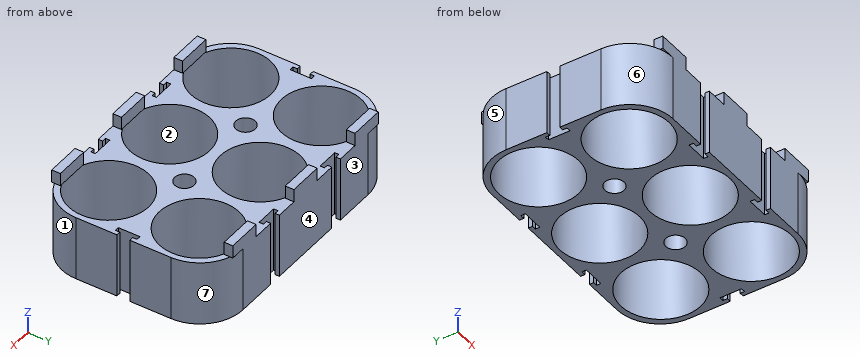
from build123d import *

# Parameters (mm, degrees)
SKETCH1_W            = 63
SKETCH1_H            = 42
SKETCH1_R            = 9.25
BOSS_EXTRUDE1_DEPTH  = 15
FILLET1_R            = 10
SKETCH3_W            = 8
SKETCH3_H            = 2
BOSS_EXTRUDE2_DEPTH  = 7
M4_CLEARANCE_HOLE1_D = 4.5
CUT_EXTRUDE1_DEPTH   = 23
SKETCH7_W            = 116.08326012
SKETCH7_H            = 87.262251834
CUT_EXTRUDE2_DEPTH   = 4


with BuildPart() as part:
    # Sketch1 → Boss-Extrude1 (new body)
    with BuildSketch(Plane.XY):
        with Locations((31.5, 21)):
            Rectangle(SKETCH1_W, SKETCH1_H)
        with Locations((10.5, 31.5)):
            Circle(SKETCH1_R, mode=Mode.SUBTRACT)
        with Locations((10.5, 10.5)):
            Circle(SKETCH1_R, mode=Mode.SUBTRACT)
        with Locations((52.5, 31.5)):
            Circle(SKETCH1_R, mode=Mode.SUBTRACT)
        with Locations((52.5, 10.5)):
            Circle(SKETCH1_R, mode=Mode.SUBTRACT)
        with Locations((31.5, 31.5)):
            Circle(SKETCH1_R, mode=Mode.SUBTRACT)
        with Locations((31.5, 10.5)):
            Circle(SKETCH1_R, mode=Mode.SUBTRACT)
    extrude(amount=BOSS_EXTRUDE1_DEPTH)

    # Fillet1
    fillet1_edges = [part.edges().sort_by_distance(p)[0] for p in [
        (0, 42, 7.5),
        (63, 42, 7.5),
        (63, 0, 7.5),
        (0, 0, 7.5),
    ]]
    fillet(fillet1_edges, radius=FILLET1_R)

    # Sketch3 → Boss-Extrude2 (add)
    with BuildSketch(Plane.XY.offset(15)):
        with Locations((31.5, 1)):
            Rectangle(SKETCH3_W, SKETCH3_H)
        with Locations((52.5, 1)):
            Rectangle(SKETCH3_W, SKETCH3_H)
        with Locations((10.5, 1)):
            Rectangle(SKETCH3_W, SKETCH3_H)
        with Locations((10.5, 41)):
            Rectangle(SKETCH3_W, SKETCH3_H)
        with Locations((31.5, 41)):
            Rectangle(SKETCH3_W, SKETCH3_H)
        with Locations((52.5, 41)):
            Rectangle(SKETCH3_W, SKETCH3_H)
    extrude(amount=BOSS_EXTRUDE2_DEPTH)

    # M4 Clearance Hole1 (through all)
    with Locations(Plane.XY.offset(15)):
        with Locations((21, 21), (42, 21)):
            Hole(M4_CLEARANCE_HOLE1_D / 2)

    # Sketch6 → Cut-Extrude1 (cut, through all)
    with BuildSketch(Plane(origin=(0, 0, 0), x_dir=(-1, 0, 0), z_dir=(0, 0, -1))):
        Polygon((-40.5, 41), (-39.5, 41), (-39.5, 40), (-44.5, 40), (-44.5, 41), (-43.5, 41), (-43.5, 42), (-40.5, 42), align=None)
        Polygon((-19.5, 41), (-18.5, 41), (-18.5, 40), (-23.5, 40), (-23.5, 41), (-22.5, 41), (-22.5, 42), (-19.5, 42), align=None)
        Polygon((-44.5, 1), (-43.5, 1), (-43.5, 0), (-40.5, 0), (-40.5, 1), (-39.5, 1), (-39.5, 2), (-44.5, 2), align=None)
        Polygon((-18.5, 2), (-18.5, 1), (-19.5, 1), (-19.5, 0), (-22.5, 0), (-22.5, 1), (-23.5, 1), (-23.5, 2), align=None)
        Polygon((-62, 19.5), (-63, 19.5), (-63, 22.5), (-62, 22.5), (-62, 23.5), (-61, 23.5), (-61, 18.5), (-62, 18.5), align=None)
        Polygon((-1, 22.5), (-1, 23.5), (-2, 23.5), (-2, 18.5), (-1, 18.5), (-1, 19.5), (0, 19.5), (0, 22.5), align=None)
    extrude(amount=-CUT_EXTRUDE1_DEPTH, mode=Mode.SUBTRACT)

    # Sketch7 → Cut-Extrude2 (cut)
    with BuildSketch(Plane.XY.offset(22)):
        with Locations((31.5, 10.5)):
            Rectangle(SKETCH7_W, SKETCH7_H)
    extrude(amount=-CUT_EXTRUDE2_DEPTH, mode=Mode.SUBTRACT)


solid = part.part
The listing builds one solid part. Answer for the finished solid, in the listing's coordinates (mm). Face numbers are marked on the shaded views. A direction names the side the tool comes from. Round coordinates to 2 decimals unless told otherwise and drop trailing zeros. Loops run counter-clockwise (first coordinate to the right, second up) from the corner with the lowest first, then second, coordinate; pieces in that order, holes last. Notation, with made-up numbers: M -18.75,27 L 1.25,27 A10 ccw 1.25,41 Z; hole C -26.75,26 d1. An arc over 180 degrees is marked long. Return JSON: item names as keys, results as strings.
Q1. The mould has two halves that part along X. Classify the marked faces 1, 2 and 3: released by +X, released by -X, zero draft, split by the parting line, or undercut.
Results list:
{"face 1": "released by +X", "face 2": "undercut", "face 3": "zero draft"}
Q2. Find section D-D, the plane y = 25. Determine the outline of the cut face in (x, z).
Results list:
{"outline": "M 0,0 L 3.92,0 L 3.92,15 L 0,15 Z; M 17.08,0 L 24.92,0 L 24.92,15 L 17.08,15 Z; M 38.08,0 L 45.92,0 L 45.92,15 L 38.08,15 Z; M 59.08,0 L 63,0 L 63,15 L 59.08,15 Z"}
Q3. Find section B-B, the plane y = 13.5. Determine the outline of the cut face in (x, z).
Results list:
{"outline": "M 0,0 L 1.75,0 L 1.75,15 L 0,15 Z; M 19.25,0 L 22.75,0 L 22.75,15 L 19.25,15 Z; M 40.25,0 L 43.75,0 L 43.75,15 L 40.25,15 Z; M 61.25,0 L 63,0 L 63,15 L 61.25,15 Z"}
Q4. Find section A-A, the plane x = 31.5. Determine the outline of the cut face in (y, z), plus the area to 3 significant figures.
Results list:
{"outline": "M 0,0 L 1.25,0 L 1.25,15 L 2,15 L 2,18 L 0,18 Z; M 19.75,0 L 22.25,0 L 22.25,15 L 19.75,15 Z; M 40,15 L 40.75,15 L 40.75,0 L 42,0 L 42,18 L 40,18 Z", "area": "87.0 mm2"}
Q5. Find section C-C, the plane x = 21. Determine the outline of the cut face in (y, z).
Results list:
{"outline": "M 2,0 L 18.75,0 L 18.75,15 L 2,15 Z; M 23.25,0 L 40,0 L 40,15 L 23.25,15 Z"}
Q6. Each of these flat-tipped pins is pushed along its axis until it touches: pin 1 Ø2 at (y, z) = (41.5, 16.5) entering from -X; pin 2 Ø1.1 at (x, z) = (61.5, 4) entering from -Y; pin 3 Ø0.6 at (y, z) = (41, 16) entering from +X. Where does it stop, or does it pass through?
Results list:
{"pin 1": "stops at x = 6.5", "pin 2": "stops at y = 3.93", "pin 3": "stops at x = 56.5"}
Q7. Find the intervals of material crossed by line 1 along Y through (x, z) = (52.5, 11.25); line 2 along X through (y, z) = (10.5, 7.5); line 3 along X through (y, z) = (20.5, 10.25), in increasing order. Write a range as from..to.
Results list:
{"line 1": "y = 0..1.25, 19.75..22.25, 40.75..42", "line 2": "x = 0..1.25, 19.75..22.25, 40.75..43.25, 61.75..63", "line 3": "x = 2..18.81, 23.19..39.81, 44.19..61"}
Q8. Which of the six approach directions +Z, -Z, +X, -X, +Y, -Y give full straight-line access (tool end or side, diameter ignored) to the marked faces 4, 5, 6 and 7?
Results list:
{"face 4": "+Z, -Z, +X, -X, +Y", "face 5": "-Z, -X, +Y", "face 6": "-Z, -X, -Y", "face 7": "-Z, +X, +Y"}
